Can you work these out from the model? Positions are in its coordinate system, mm. A direction names the side the tool comes from. Coordinates: 2 decimals unless noted, no trailing zeros. Loops run counter-clockwise (first coordinate to the right, second up) from the corner with the lowest first, then second, coordinate; pieces in that order, holes last. Notation, with made-up numbers: (-21, 37.25) -> (33, 37.25) arc R22 ccw to (33, 65.25) -> close; hole circle Ø2 at (76.5, 74.5). An arc over 180 degrees is marked (long way). Put each result on its own line as item: value. Start each with the question number.
Item 1: If we section it at A-A on y = 23.5: Please give me the cut outline in (x, z), plus the area to 3 significant figures.
Item 2: If we section it at D-D on z = 45.5: Please give me the cut outline in (x, y), plus the area to 3 significant figures.
Item 3: We'd pull the mould along Z, two halves only. Please class faces 1 (the flat face through (13, -27.5, 2)), 2 (the cylindrical face through (0.14, -46.93, 0.6)), 3 (the cylindrical face through (0.14, -42.9, 43.43)), 4 (the cylindrical face through (0.14, -46.9, 53.43)): pulls with the +Z half, pulls with the -Z half, needs draft (parallel to the pull), parting line crosses it, or undercut.
Item 4: Please list where these lines run through material, in increasing order: L1, parallel to Z at x = -15, y = -19; L2, parallel to Y at x = -15.5, z = 2.35; L3, parallel to X at y = -15, z = 2. Write a range as from..to.
Item 5: If we section it at C-C on y = 15.5: Please give me the cut outline in (x, z).
Item 6: Will these pins go through, and if not, where does the flat tip stop? P1, Ø20, axis at x = 0, y = 0, coming from the -Z side; P2, Ø14.5, axis at y = -38.5, z = 24.5, coming from the +X side; P3, Ø8, axis at x = 0, z = 14, coming from the +Y side.
Item 7: For faces 5 (the flat face through (-14, -27.5, 49)), 6 (the flat face through (10, -45, 33)), 7 (the flat face through (0, -7, 44)), which set-ups out of +Z, -Z, +X, -X, +Y, -Y let a thin tool reach every point of the face, with its end or its side?
Item 8: If we section it at B-B on z = 34: Please give me the cut outline in (x, y), plus the area to 3 significant figures.
```python
from build123d import *

# Parameters (mm, degrees)
SCHIZZO1_R                   = 1.75
SCHIZZO1_R_2                 = 11.05
ESTRUSIONE_ESTRUSIONE1_DEPTH = 4
SCHIZZO14_W                  = 20
SCHIZZO14_H                  = 4
ESTRUSIONE_ESTRUSIONE2_DEPTH = 40
ESTRUSIONE_ESTRUSIONE3_DEPTH = 10
SCHIZZO19_R                  = 11
TAGLIO_ESTRUSIONE1_DEPTH     = 7
SCHIZZO20_R                  = 4
TAGLIO_ESTRUSIONE2_DEPTH     = 7
SMUSSO1_SIZE                 = 10
RACCORDO1_R                  = 2
SCHIZZO21_R                  = 2.5
TAGLIO_ESTRUSIONE3_DEPTH     = 10


with BuildPart() as part:
    # Schizzo1 → Estrusione-Estrusione1 (new body)
    with BuildSketch(Plane.XY):
        Polygon((-25, -27.5), (-10, -27.5), (-10, -47.5), (10, -47.5), (10, -27.5), (25, -27.5), (25, 27.5), (-25, 27.5), align=None)
        with Locations((-15.5, 15.5)):
            Circle(SCHIZZO1_R, mode=Mode.SUBTRACT)
        with Locations((15.5, 15.5)):
            Circle(SCHIZZO1_R, mode=Mode.SUBTRACT)
        with Locations((15.5, -15.5)):
            Circle(SCHIZZO1_R, mode=Mode.SUBTRACT)
        with Locations((-15.5, -15.5)):
            Circle(SCHIZZO1_R, mode=Mode.SUBTRACT)
        Circle(SCHIZZO1_R_2, mode=Mode.SUBTRACT)
    extrude(amount=ESTRUSIONE_ESTRUSIONE1_DEPTH)

    # Schizzo14 → Estrusione-Estrusione2 (add)
    with BuildSketch(Plane.XY.offset(4)):
        with Locations((0, -45.5)):
            Rectangle(SCHIZZO14_W, SCHIZZO14_H)
    extrude(amount=ESTRUSIONE_ESTRUSIONE2_DEPTH)

    # Schizzo18 → Estrusione-Estrusione3 (add)
    with BuildSketch(Plane.XY.offset(44)):
        Polygon((-25, -27.5), (-10, -27.5), (-10, -47.5), (10, -47.5), (10, -27.5), (25, -27.5), (25, 27.5), (-25, 27.5), align=None)
    extrude(amount=ESTRUSIONE_ESTRUSIONE3_DEPTH)

    # Schizzo19 → Taglio-Estrusione1 (cut)
    with BuildSketch(Plane.XY.offset(54)):
        Circle(SCHIZZO19_R)
    extrude(amount=-TAGLIO_ESTRUSIONE1_DEPTH, mode=Mode.SUBTRACT)

    # Schizzo20 → Taglio-Estrusione2 (cut)
    with BuildSketch(Plane.XY.offset(47)):
        Circle(SCHIZZO20_R)
    extrude(amount=-TAGLIO_ESTRUSIONE2_DEPTH, mode=Mode.SUBTRACT)

    # Smusso1
    smusso1_edges = [part.edges().sort_by_distance(p)[0] for p in [
        (25, -27.5, 2),
        (-25, -27.5, 2),
        (-25, 27.5, 2),
        (25, 27.5, 2),
        (25, -27.5, 49),
        (25, 27.5, 49),
        (-25, 27.5, 49),
        (-25, -27.5, 49),
    ]]
    chamfer(smusso1_edges, length=SMUSSO1_SIZE)

    # Raccordo1
    raccordo1_edges = [part.edges().sort_by_distance(p)[0] for p in [
        (10, -27.5, 2),
        (-10, -27.5, 2),
        (0, -43.5, 4),
        (0, -43.5, 44),
        (-10, -27.5, 49),
        (10, -27.5, 49),
        (0, -47.5, 54),
        (0, -47.5, 0),
    ]]
    fillet(raccordo1_edges, radius=RACCORDO1_R)

    # Schizzo21 → Taglio-Estrusione3 (cut)
    with BuildSketch(Plane(origin=(0, -43.5, 0), x_dir=(1, 0, 0), z_dir=(0, 1, 0))):
        with Locations((0, -14)):
            Circle(SCHIZZO21_R)
        with Locations((0, -34)):
            Circle(SCHIZZO21_R)
    extrude(amount=-TAGLIO_ESTRUSIONE3_DEPTH, mode=Mode.SUBTRACT)


solid = part.part
```
Solutions:
1. outline: (-19, 0) -> (19, 0) -> (19, 4) -> (-19, 4) -> close; (-19, 44) -> (19, 44) -> (19, 54) -> (-19, 54) -> close
1. area: 532 mm^2
2. outline: (-25, -17.5) -> (-15, -27.5) -> (-12, -27.5) arc R2 cw to (-10, -29.5) -> (-10, -47.5) -> (10, -47.5) -> (10, -29.5) arc R2 cw to (12, -27.5) -> (15, -27.5) -> (25, -17.5) -> (25, 17.5) -> (15, 27.5) -> (-15, 27.5) -> (-25, 17.5) -> close; hole circle Ø8 at (0, 0)
2. area: 2,900 mm^2
3. face 1: needs draft
3. face 2: pulls with the -Z half
3. face 3: undercut
3. face 4: pulls with the +Z half
4. L1: 0..4, 44..54
4. L2: -27..-17.25, -13.75..13.75, 17.25..27
4. L3: -25..-17.18, -13.82..13.82, 17.18..25
5. outline: (-25, 0) -> (-17.25, 0) -> (-17.25, 4) -> (-25, 4) -> close; (-25, 44) -> (25, 44) -> (25, 54) -> (-25, 54) -> close; (-13.75, 0) -> (13.75, 0) -> (13.75, 4) -> (-13.75, 4) -> close; (17.25, 0) -> (25, 0) -> (25, 4) -> (17.25, 4) -> close
6. P1: z = 44
6. P2: x = 10
6. P3: y = -43.5
7. face 5: +Z, -Z, -X, -Y
7. face 6: +Z, -Z, +X, -Y
7. face 7: +X, -X, +Y
8. outline: (-10, -47.5) -> (-2.5, -47.5) -> (-2.5, -43.5) -> (-10, -43.5) -> close; (2.5, -47.5) -> (10, -47.5) -> (10, -43.5) -> (2.5, -43.5) -> close
8. area: 60.0 mm^2
